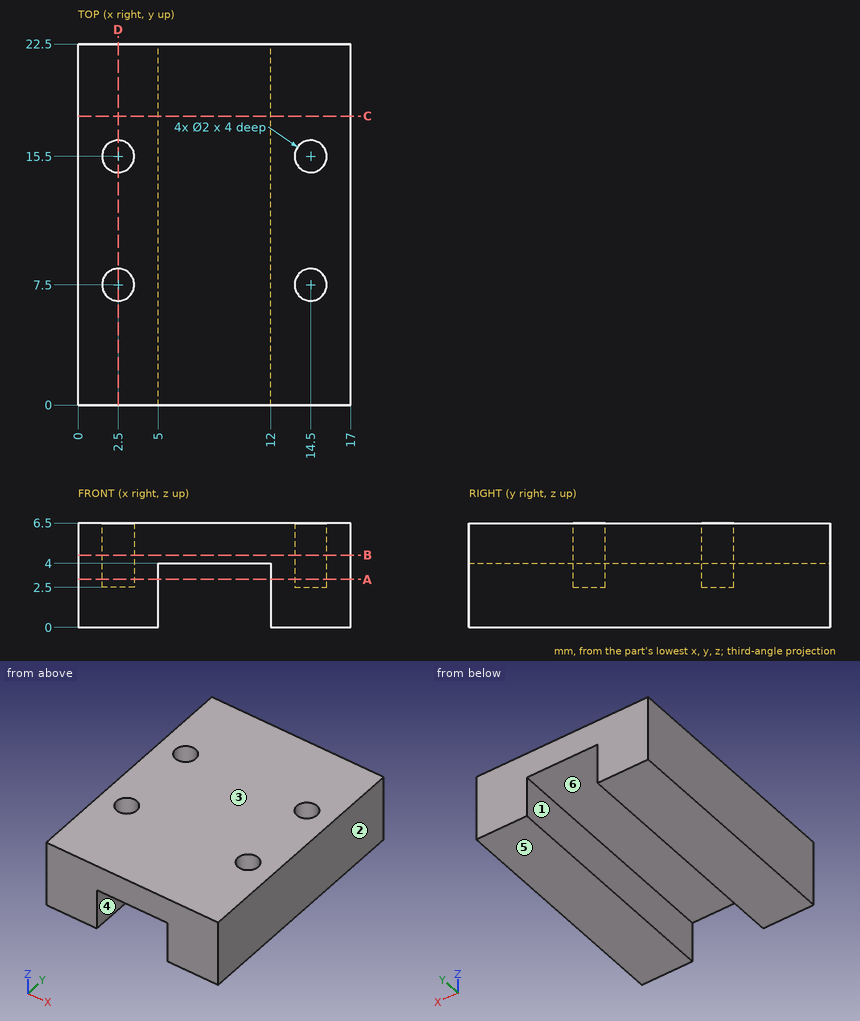
Verification items for this drawing (mm, ordinates from the low corner). A direction names the side the tool comes from. Coordinates: 2 decimals unless noted, no trailing zeros. Write each loop counter-clockwise with the first axis right and the second up, starting at its lowest first coordinate (ties: lowest second). Pieces come first, ordered by that corner, then holes. Notation, with made-up numbers: M 34.5,62.5 L 92.5,62.5 A30 cw 92.5,95.5 Z; hole C 23.5,-27.5 d8. An arc over 180 degrees is marked long. Answer as a JSON object with one key per item and string values.
1. Go/stop test with a flat-tipped pin: pin 1 Ø2 at (x, y) = (8.5, 14.5) entering from -Z. Record where the tip stops, or that it passes through.
Answers below:
{"pin 1": "stops at z = 4"}
2. Scan lines: L1, parallel to Y at x = 14.5, z = 4.9; L2, parallel to X at y = 16.75, z = 2; L3, parallel to Z at x = 3, y = 6.75. Record each from-to range of solid material in increasing order.
Answers below:
{"L1": "y = 0 to 6.5, 8.5 to 14.5, 16.5 to 22.5", "L2": "x = 0 to 5, 12 to 17", "L3": "z = 0 to 2.5"}
3. Section check A-A, the plane z = 3. Enter the section's corners in (x, y), plus the area to 3 significant figures.
Answers below:
{"outline": "M 0,0 L 5,0 L 5,22.5 L 0,22.5 Z; M 12,0 L 17,0 L 17,22.5 L 12,22.5 Z; hole C 2.5,7.5 d2; hole C 2.5,15.5 d2; hole C 14.5,7.5 d2; hole C 14.5,15.5 d2", "area": "212 mm²"}
4. Section check D-D, the plane x = 2.5. Enter the section's corners in (y, z).
Answers below:
{"outline": "M 0,0 L 22.5,0 L 22.5,6.5 L 16.5,6.5 L 16.5,2.5 L 14.5,2.5 L 14.5,6.5 L 8.5,6.5 L 8.5,2.5 L 6.5,2.5 L 6.5,6.5 L 0,6.5 Z"}
5. Section check C-C, the plane y = 18. Enter the section's corners in (x, z).
Answers below:
{"outline": "M 0,0 L 5,0 L 5,4 L 12,4 L 12,0 L 17,0 L 17,6.5 L 0,6.5 Z"}
6. Section check B-B, the plane z = 4.5. Enter the section's corners in (x, y), plus the area to 3 significant figures.
Answers below:
{"outline": "M 0,0 L 17,0 L 17,22.5 L 0,22.5 Z; hole C 2.5,7.5 d2; hole C 2.5,15.5 d2; hole C 14.5,7.5 d2; hole C 14.5,15.5 d2", "area": "370 mm²"}
7. Tool access check on the marked faces 5 and 6. Record the directions out of +Z, -Z, +X, -X, +Y, -Y that give a thin tool (end or side, any length) a straight path to the whole face; none if there is none.
Answers below:
{"face 5": "-Z, +X, -X, +Y, -Y", "face 6": "-Z, +Y, -Y"}
8. Draft check along X on the marked faces 1, 2, 3 and 4. Enter one of: released by +X, released by -X, zero draft, split by the parting line, or undercut.
Answers below:
{"face 1": "undercut", "face 2": "released by +X", "face 3": "zero draft", "face 4": "undercut"}
